Design review of the part shown in the three views and the two pictorial views. Dimensions are in mm from the part's minimum x, y and z. A direction names the side the tool comes from. Give positions to 0.01 mm unless a question says otherwise; leave off trailing zeros. Loops run counter-clockwise (first coordinate to the right, second up) from the corner with the lowest first, then second, coordinate; pieces in that order, holes last. Notation, with made-up numbers: (55, 30.25) -> (91, 30.25) arc R14 ccw to (91, 41.25) -> close; hole circle Ø9 at (-6.75, -13.5). An arc over 180 degrees is marked (long way). One line per question, with ' | ' between items. Start each with the question number.
(1) Consider section A-A (y = 37). Write out the cut boundary in (x, z) (1 decimal).
(2) Tool access review of the marked faces 1, 2 and 3: name each direction out of +Z, -Z, +X, -X, +Y, -Y from which nothing blocks a thin tool from reaching the whole face with its end or side.
(3) Wall thickness on probe 1 along Y at (x, z) = (27, 40.5); probe 2 along Z at (x, y) = (22, 48) (1 decimal); probe 3 along X at (y, z) = (73, 27) (1 decimal): over which ranges is each line inside the solid? List them lowest first.
(4) Consider section B-B (y = 170.5). Write out the cut boundary in (x, z).
(5) Insertion check: P1, Ø17.5, axis at x = 23.5, y = 83, coming from the +Z side; P2, Ø1.5, axis at x = 24, z = 6.5, coming from the -Y side; P3, Ø8, axis at y = 152, z = 24.5, coming from the +X side. Each pin has a flat end and moves straight along its axis. Give the tip position at first contact, or say it passes through.
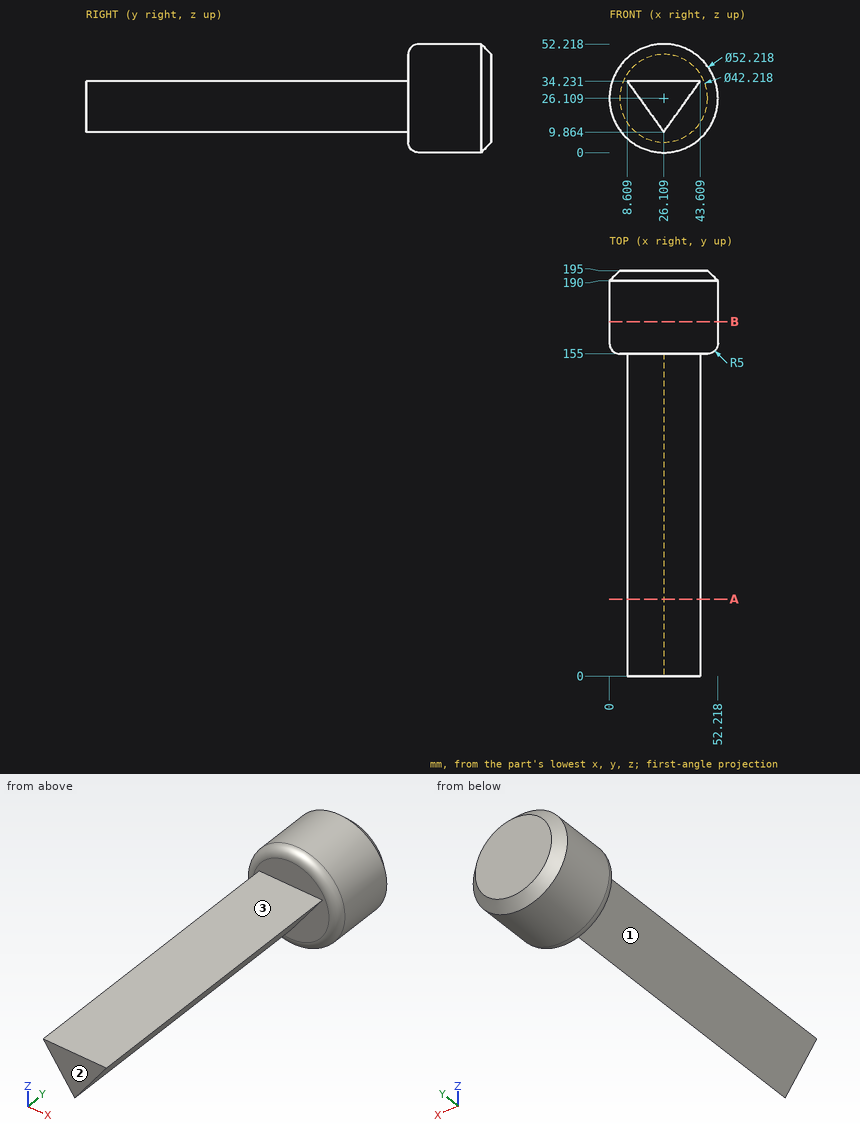
A:
1) outline: (8.6, 34.2) -> (26.1, 9.9) -> (43.6, 34.2) -> close
2) face 1: -Z, -X, -Y | face 2: +Z, -Z, +X, -X, -Y | face 3: +Z, +X, -X, -Y
3) probe 1: y = 155 to 195 | probe 2: z = 15.6 to 34.2 | probe 3: x = 13.8 to 38.4
4) outline: circle Ø52.22 at (26.11, 26.11)
5) P1: stops at z = 34.23 | P2: stops at y = 155 | P3: stops at x = 50.17
